Read the model definition and answer for the solid it produces. Units are mm, in the model's axes. A direction names the side the tool comes from. Give positions to 0.01 mm unless a question says otherwise; leave off trailing zeros. Loops run counter-clockwise (first coordinate to the right, second up) from the corner with the lowest first, then second, coordinate; pieces in that order, holes last. Notation, with made-up numbers: (42, 23) -> (57, 23) arc R19 ccw to (57, 56) -> close; hole circle Ø3 at (80.25, 42). An arc over 180 degrees is marked (long way). Answer as CSV lines item,"result". Start each with the question number.
```python
from build123d import *

# Parameters (mm, degrees)
CYLINDER_R              = 100
CYLINDER_DEPTH          = 400
CYLINDER_PITCH_ANGLE    = 45
CYLINDER001_R           = 105
CYLINDER001_DEPTH       = 400
CYLINDER001_PITCH_ANGLE = 45


with BuildPart() as cylinder:
    # Cylinder → Cylinder (new body)
    with BuildSketch(Plane.XY):
        Circle(CYLINDER_R)
    extrude(amount=CYLINDER_DEPTH)


with BuildPart() as cylinder_1:
    # Cylinder pitch: moved
    add(cylinder.part.rotate(Axis((0, 0, 0), (0, 1, 0)), CYLINDER_PITCH_ANGLE))


with BuildPart() as cylinder_2:
    # Cylinder placement: moved
    add(cylinder_1.part.moved(Location((99.702056, 0, 99.702056))))


with BuildPart() as fusion:
    # Cone → Cone (revolve)
    with BuildSketch(Plane.XZ):
        Polygon((0, 0), (200, 0), (100, 400), (0, 400), align=None)
    revolve(axis=Axis((0, 0, 0), (0, 0, 1)))

    # Fusion: union Cylinder
    add(cylinder_2.part)


with BuildPart() as cylinder001:
    # Cylinder001 → Cylinder001 (new body)
    with BuildSketch(Plane.XY):
        Circle(CYLINDER001_R)
    extrude(amount=CYLINDER001_DEPTH)


with BuildPart() as cylinder001_1:
    # Cylinder001 pitch: moved
    add(cylinder001.part.rotate(Axis((0, 0, 0), (0, 1, 0)), CYLINDER001_PITCH_ANGLE))


with BuildPart() as cylinder001_2:
    # Cylinder001 placement: moved
    add(cylinder001_1.part.moved(Location((99.702056, 0, 99.702056))))


with BuildPart() as cut:
    # Cone001 → Cone001 (revolve)
    with BuildSketch(Plane.XZ):
        Polygon((0, 0), (205, 0), (105, 400), (0, 400), align=None)
    revolve(axis=Axis((0, 0, 0), (0, 0, 1)))

    # Fusion001: union Cylinder001
    add(cylinder001_2.part)

    # Cut: cut Fusion
    add(fusion.part, mode=Mode.SUBTRACT)


solid = cut.part
```
(1) The mould has two halves that part along Y. Classify faces 1 (the face through (319.961, 31.539, 178.326)), 2 (the face through (313.523, -38.301, 182.885)), 3 (the face through (-196, -45, 0)), 4 (the face through (-138.055, 6.076, 247.244)): pulls with the +Y half, pulls with the -Y half, needs draft (parallel to the pull), parting line crosses it, or undercut.
(2) Find section C-C on y = 57. Give the number of separate pieces and of enclosed holes in the cut face, then the cut area to 3 significant figures.
(3) Find the intervals of material crossed by line 1 along X through (y, z) = (44, 322.5); line 2 along X through (y, z) = (53.5, 285); line 3 along Y through (x, z) = (111, 158), in increasing order. Write a range as from..to.
(4) Find section B-B on y = 0. Write down the section's boundary in (x, z), then the cut area to 3 significant figures.
(5) Find section A-A on x = 0. Write down the section's boundary in (y, z), then the cut area to 3 significant figures.
(6) Each of these flat-tipped pins is pushed along its axis until it touches: P1, Ø12, axis at x = -138, z = 74.5, coming from the +Y side; P2, Ø6, axis at x = 7.5, z = 261.5, coming from the -Y side; P3, Ø3, axis at x = 101.5, z = 267, coming from the -Y side. Where does it stop, or does it pass through?
(7) A tool of negligible diameter and unlimited length cuts with its end or side. For faces 5 (the face through (409.7, -92.84, 355.39)), 6 (the face through (93, -38, 400)), from which of +Z, -Z, +X, -X, +Y, -Y can it reach the whole face along a straight path? Write none if from no direction.
Answer block:
1,face 1,"parting line crosses it"
1,face 2,"undercut"
1,face 3,"needs draft"
1,face 4,"undercut"
2,separate pieces,"3"
2,enclosed holes,"0"
2,area,"7,250 mm2"
3,line 1,"x = -116.33..-110.97, 110.97..116.33, 187.67..195.5"
3,line 2,"x = -122.58..-117.11, 117.11..122.58, 157.23..165.52, 404.48..412.77"
3,line 3,"y = -122.76..-115.93, 115.93..122.76"
4,outline,"(-205, 0) -> (-200, 0) -> (-100, 400) -> (-105, 400) -> close; (100, 400) -> (131.72, 273.14) -> (311.83, 453.26) -> (308.3, 456.79) -> (134.3, 282.79) -> (105, 400) -> close; (188.28, 46.86) -> (200, 0) -> (205, 0) -> (193.7, 45.21) -> (456.79, 308.3) -> (453.26, 311.83) -> close"
4,area,"5,960 mm2"
5,outline,"(-205, 0) -> (-200, 0) -> (-100, 400) -> (-105, 400) -> close; (100, 400) -> (200, 0) -> (205, 0) -> (105, 400) -> close"
5,area,"4,000 mm2"
6,P1,"stops at y = 131.94"
6,P2,"stops at y = -140.19"
6,P3,"stops at y = -95.55"
7,face 5,"+Z, +X, +Y, -Y"
7,face 6,"+Z, -X, +Y, -Y"
